Design review of the part built by this model. Coordinates are the model's own, in mm. Give positions to 0.01 mm unless a question says otherwise; leave off trailing zeros. Write each loop counter-clockwise with the first axis right and the second up, starting at its lowest first coordinate (ties: lowest second). Pieces come first, ordered by that corner, then holes.
```python
from build123d import *

# Parameters (mm, degrees)
EXTRUDE_1_DEPTH     = 3.2
SKETCH_2_W          = 28
SKETCH_2_H          = 3
CUT_EXTRUDE_1_DEPTH = 2
SKETCH_3_W          = 5
SKETCH_3_H          = 12
EXTRUDE_2_DEPTH     = 7
SKETCH_4_R          = 1
CUT_EXTRUDE_2_DEPTH = 243.070789578


with BuildPart() as part:
    # 草图1 → 凸台-拉伸1 (new body)
    with BuildSketch(Plane.XY):
        with BuildLine():
            Line((-107.202531646, -47.623114492), (64.797468354, -47.623114492))
            Line((64.797468354, -47.623114492), (64.797468354, -50.623114492))
            Line((64.797468354, -50.623114492), (92.797468354, -50.623114492))
            Line((92.797468354, -50.623114492), (92.797468354, -47.623114492))
            Line((92.797468354, -47.623114492), (123.797468354, -47.623114492))
            Line((123.797468354, -47.623114492), (123.797468354, 62.376885508))
            ThreePointArc((123.797468354, 62.376885508), (120.868536166, 69.447953319), (113.797468354, 72.376885508))
            Line((113.797468354, 72.376885508), (-156.202531646, 72.376885508))
            ThreePointArc((-156.202531646, 72.376885508), (-163.273599457, 69.447953319), (-166.202531646, 62.376885508))
            Line((-166.202531646, 62.376885508), (-166.202531646, -47.623114492))
            Line((-166.202531646, -47.623114492), (-135.202531646, -47.623114492))
            Line((-135.202531646, -47.623114492), (-135.202531646, -50.623114492))
            Line((-135.202531646, -50.623114492), (-107.202531646, -50.623114492))
            Line((-107.202531646, -50.623114492), (-107.202531646, -47.623114492))
        make_face()
    extrude(amount=EXTRUDE_1_DEPTH)

    # 草图2 → 切除-拉伸1 (cut)
    with BuildSketch(Plane.XY.offset(3.2)):
        with Locations((-121.202531646, -49.123114492)):
            Rectangle(SKETCH_2_W, SKETCH_2_H)
        with Locations((78.797468354, -49.123114492)):
            Rectangle(SKETCH_2_W, SKETCH_2_H)
    extrude(amount=-CUT_EXTRUDE_1_DEPTH, mode=Mode.SUBTRACT)

    # 草图3 → 凸台-拉伸2 (add)
    with BuildSketch(Plane.XY):
        with Locations((-129.902531646, 13.376885508)):
            Rectangle(SKETCH_3_W, SKETCH_3_H)
        with Locations((87.497468354, 13.376885508)):
            Rectangle(SKETCH_3_W, SKETCH_3_H)
    extrude(amount=-EXTRUDE_2_DEPTH)

    # 草图4 → 切除-拉伸2 (cut, through all)
    with BuildSketch(Plane(origin=(65.420582847, 19.376885508, 0), x_dir=(0, 0, -1), z_dir=(0, -1, 0))):
        with Locations(Location((4.5, -195.323114492, 0), (0, 0, 90))):
            Circle(SKETCH_4_R)
        with Locations(Location((4.5, 22.076885508, 0), (0, 0, 90))):
            Circle(SKETCH_4_R)
    extrude(amount=CUT_EXTRUDE_2_DEPTH, mode=Mode.SUBTRACT)


solid = part.part
```
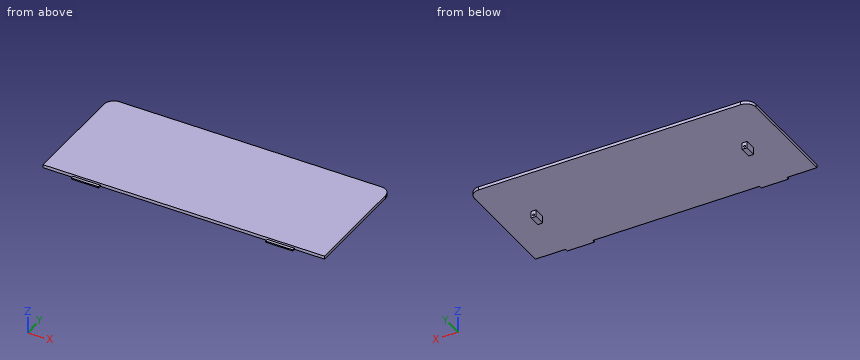
(1) Consider section C-C, the plane y = -38. Give the boundary of the cut face in (x, z), then the cut area to 3 significant figures.
Resolved:
outline: (-166.2, 0) - (123.8, 0) - (123.8, 3.2) - (-166.2, 3.2) - close
area: 928 mm2
(2) Consider section B-B, the plane x = -110.5. Give the boundary of the cut face in (y, z), then the cut area to 3 significant figures.
Resolved:
outline: (-50.62, 0) - (72.38, 0) - (72.38, 3.2) - (-47.62, 3.2) - (-47.62, 1.2) - (-50.62, 1.2) - close
area: 388 mm2
(3) To check wall thickness, follow L1, parallel to X at y = 13.5, z = -4.5; L2, parallel to Z at x = -54.5, y = -12; L3, parallel to Y at x = 23, z = 1. State the ranges of each line that lie inside material, in increasing order.
Resolved:
L1: x = -132.4 to -130.9, -128.9 to -127.4, 85 to 86.5, 88.5 to 90
L2: z = 0 to 3.2
L3: y = -47.62 to 72.38
(4) Consider section A-A, the plane y = 16. Give the boundary of the cut face in (x, z).
Resolved:
outline: (-166.2, 0) - (-132.4, 0) - (-132.4, -7) - (-127.4, -7) - (-127.4, 0) - (85, 0) - (85, -7) - (90, -7) - (90, 0) - (123.8, 0) - (123.8, 3.2) - (-166.2, 3.2) - close; hole circle Ø2 at (-129.9, -4.5); hole circle Ø2 at (87.5, -4.5)
(5) Clearance check with flat-ended pins moving along their axes: P1, Ø3.5, axis at y = 16, z = -4, coming from the +X side; P2, Ø1.5, axis at x = -81, y = 42.5, coming from the -Z side; P3, Ø0.9, axis at x = 84, y = -48.5, coming from the +Z side. State where each tip first meets the part, or that it passes through.
Resolved:
P1: stops at x = 90
P2: stops at z = 0
P3: stops at z = 1.2
(6) Consider section D-D, the plane x = 100. Give the boundary of the cut face in (y, z).
Resolved:
outline: (-47.62, 0) - (72.38, 0) - (72.38, 3.2) - (-47.62, 3.2) - close
